from build123d import *

# Parameters (mm, degrees)
SKETCH1_W           = 102
SKETCH1_H           = 85
BOSS_EXTRUDE1_DEPTH = 38
SKETCH2_R           = 2.1
CUT_EXTRUDE1_DEPTH  = 35
SKETCH3_R           = 2.1
CUT_EXTRUDE2_DEPTH  = 35
SKETCH5_R           = 4
CUT_EXTRUDE4_DEPTH  = 10
FILLET1_R           = 5
FILLET2_R           = 5
FILLET3_R           = 5
FILLET4_R           = 5
SKETCH6_R           = 1.6
BOSS_EXTRUDE2_DEPTH = 5
SKETCH7_W           = 15
SKETCH7_H           = 4
BOSS_EXTRUDE3_DEPTH = 12
CHAMFER1_SIZE       = 5
CHAMFER2_SIZE       = 5
SKETCH8_R           = 3.012300636
CUT_EXTRUDE5_DEPTH  = 5
FILLET5_R           = 2
FILLET6_R           = 2
FILLET7_R           = 2
FILLET8_R           = 2
SKETCH9_W           = 1
SKETCH9_H           = 10
CUT_EXTRUDE6_DEPTH  = 2.1
SKETCH10_W          = 1
SKETCH10_H          = 10
CUT_EXTRUDE7_DEPTH  = 2.1


with BuildPart() as part:
    # Sketch1 → Boss-Extrude1 (new body)
    with BuildSketch(Plane(origin=(0, 0, 0), x_dir=(1, 0, 0), z_dir=(0, 1, 0))):
        Rectangle(SKETCH1_W, SKETCH1_H)
    extrude(amount=BOSS_EXTRUDE1_DEPTH)

    # Sketch2 → Cut-Extrude1 (cut)
    with BuildSketch(Plane(origin=(0, 38, 0), x_dir=(1, 0, 0), z_dir=(0, 1, 0))):
        with Locations((43, 34.5)):
            Circle(SKETCH2_R)
        with Locations((-43, -34.5)):
            Circle(SKETCH2_R)
        with Locations((43, -34.5)):
            Circle(SKETCH2_R)
        Polygon((-39, 40.5), (39, 40.5), (39, 30.5), (49, 30.5), (49, -30.5), (39, -30.5), (39, -40.5), (-39, -40.5), (-39, -30.5), (-49, -30.5), (-49, 30.5), (-39, 30.5), align=None)
    extrude(amount=-CUT_EXTRUDE1_DEPTH, mode=Mode.SUBTRACT)

    # Sketch3 → Cut-Extrude2 (cut)
    with BuildSketch(Plane(origin=(0, 38, 0), x_dir=(1, 0, 0), z_dir=(0, 1, 0))):
        with Locations((-43, 34.5)):
            Circle(SKETCH3_R)
    extrude(amount=-CUT_EXTRUDE2_DEPTH, mode=Mode.SUBTRACT)

    # Sketch5 → Cut-Extrude4 (cut)
    with BuildSketch(Plane.ZY.offset(51)):
        with Locations((-17.5, 7.998461061)):
            Circle(SKETCH5_R)
        with Locations((17.5, 7.998461061)):
            Circle(SKETCH5_R)
    extrude(amount=-CUT_EXTRUDE4_DEPTH, mode=Mode.SUBTRACT)

    # Fillet1
    fillet1_edges = [part.edges().sort_by_distance(p)[0] for p in [
        (-51, 19, 42.5),
    ]]
    fillet(fillet1_edges, radius=FILLET1_R)

    # Fillet2
    fillet2_edges = [part.edges().sort_by_distance(p)[0] for p in [
        (-51, 19, -42.5),
    ]]
    fillet(fillet2_edges, radius=FILLET2_R)

    # Fillet3
    fillet3_edges = [part.edges().sort_by_distance(p)[0] for p in [
        (51, 19, 42.5),
    ]]
    fillet(fillet3_edges, radius=FILLET3_R)

    # Fillet4
    fillet4_edges = [part.edges().sort_by_distance(p)[0] for p in [
        (51, 19, -42.5),
    ]]
    fillet(fillet4_edges, radius=FILLET4_R)

    # Sketch6 → Boss-Extrude2 (add)
    with BuildSketch(Plane(origin=(0, 3, 0), x_dir=(1, 0, 0), z_dir=(0, 1, 0))):
        with Locations((-33.5, 26.565019739)):
            Circle(SKETCH6_R)
        with Locations((-33.5, -5.434980261)):
            Circle(SKETCH6_R)
        with Locations((33.5, 26.565019739)):
            Circle(SKETCH6_R)
        with Locations((33.5, -5.434980261)):
            Circle(SKETCH6_R)
    extrude(amount=BOSS_EXTRUDE2_DEPTH)

    # Sketch7 → Boss-Extrude3 (add)
    with BuildSketch(Plane.ZY.offset(51)):
        with Locations((0, 2)):
            Rectangle(SKETCH7_W, SKETCH7_H)
    extrude(amount=BOSS_EXTRUDE3_DEPTH)

    # Chamfer1
    chamfer1_edges = [part.edges().sort_by_distance(p)[0] for p in [
        (-63, 2, -7.5),
    ]]
    chamfer(chamfer1_edges, length=CHAMFER1_SIZE)

    # Chamfer2
    chamfer2_edges = [part.edges().sort_by_distance(p)[0] for p in [
        (-63, 2, 7.5),
    ]]
    chamfer(chamfer2_edges, length=CHAMFER2_SIZE)

    # Sketch8 → Cut-Extrude5 (cut)
    with BuildSketch(Plane(origin=(0, 4, 0), x_dir=(1, 0, 0), z_dir=(0, 1, 0))):
        with Locations((-56.61368814, 0)):
            Circle(SKETCH8_R)
    extrude(amount=-CUT_EXTRUDE5_DEPTH, mode=Mode.SUBTRACT)

    # Fillet5
    fillet5_edges = [part.edges().sort_by_distance(p)[0] for p in [
        (-58, 2, -7.5),
    ]]
    fillet(fillet5_edges, radius=FILLET5_R)

    # Fillet6
    fillet6_edges = [part.edges().sort_by_distance(p)[0] for p in [
        (-63, 2, -2.5),
    ]]
    fillet(fillet6_edges, radius=FILLET6_R)

    # Fillet7
    fillet7_edges = [part.edges().sort_by_distance(p)[0] for p in [
        (-63, 2, 2.5),
    ]]
    fillet(fillet7_edges, radius=FILLET7_R)

    # Fillet8
    fillet8_edges = [part.edges().sort_by_distance(p)[0] for p in [
        (-58, 2, 7.5),
    ]]
    fillet(fillet8_edges, radius=FILLET8_R)

    # Sketch9 → Cut-Extrude6 (cut)
    with BuildSketch(Plane.XY.offset(42.5)):
        with Locations((-30.5, 28)):
            Rectangle(SKETCH9_W, SKETCH9_H)
    extrude(amount=-CUT_EXTRUDE6_DEPTH, mode=Mode.SUBTRACT)

    # Sketch10 → Cut-Extrude7 (cut)
    with BuildSketch(Plane.XY.offset(42.5)):
        with Locations((-27.5, 28)):
            Rectangle(SKETCH10_W, SKETCH10_H)
        with Locations((-24.5, 28)):
            Rectangle(SKETCH10_W, SKETCH10_H)
        with Locations((-21.5, 28)):
            Rectangle(SKETCH10_W, SKETCH10_H)
    extrude(amount=-CUT_EXTRUDE7_DEPTH, mode=Mode.SUBTRACT)


solid = part.part
Check sheet for the modelled part. Datum: model origin and axes. Units: mm. A direction names the side the tool comes from. Round coordinates to 2 decimals unless told otherwise and drop trailing zeros. Loops run counter-clockwise (first coordinate to the right, second up) from the corner with the lowest first, then second, coordinate; pieces in that order, holes last.
1. Sectioned sample at D-D on z = 34.5. Record the boundary of the cut face in (x, y).
2. Sectioned sample at C-C on x = -33.5. Record the boundary of the cut face in (y, z).
3. Sectioned sample at B-B on y = 18.5. Record the boundary of the cut face in (x, z), and give its area (3 significant figures).
4. Gauge pin test, flat ends, axial feed: pin 1 Ø3.5 at (x, z) = (-56.5, 0) entering from +Y; pin 2 Ø1.6 at (y, z) = (28, 41.5) entering from +X; pin 3 Ø2 at (x, z) = (-23, 3) entering from -Y; pin 4 Ø1 at (y, z) = (32, -26.5) entering from -X. Record the tip position at first contact, or that the pin passes through.
5. Sectioned sample at A-A on z = 17.5. Record the boundary of the cut face in (x, y).
6. Mould release check, pull along X, two halves, no side actions. Record for faces 4 (the flat face through (-43, 3, -35)), 5 (the flat face through (-63, 2, 0)), 6 (the flat face through (-49.3, 38, -0.2)): released by +X, released by -X, zero draft, split by the parting line, or undercut.
7. Scan lines: probe 1 along Z at (x, y) = (-43, 22); probe 2 along X at (y, z) = (26, 34.5); probe 3 along Z at (x, y) = (19, 8). Record each from-to range of solid material in increasing order.
8. Set-up check for faces 1 (the flat face through (-60.5, 2, 5)), 2 (the flat face through (-44, 21, -30.5)), 3 (the cylindrical face through (-50.014, 8.174, -21.496)): record each of +Z, -Z, +X, -X, +Y, -Y from which the full face is reachable in a straight line by a thin tool's end or side.
Recorded:
1. outline: (-51, 0) - (51, 0) - (51, 38) - (45.1, 38) - (45.1, 3) - (40.9, 3) - (40.9, 38) - (39, 38) - (39, 3) - (-39, 3) - (-39, 38) - (-40.9, 38) - (-40.9, 3) - (-45.1, 3) - (-45.1, 38) - (-51, 38) - close
2. outline: (0, -42.5) - (38, -42.5) - (38, -40.5) - (3, -40.5) - (3, -28.17) - (8, -28.17) - (8, -24.97) - (3, -24.97) - (3, 3.83) - (8, 3.83) - (8, 7.03) - (3, 7.03) - (3, 40.5) - (38, 40.5) - (38, 42.5) - (0, 42.5) - close
3. outline: (-51, -37.5) arc R5 ccw to (-46, -42.5) - (46, -42.5) arc R5 ccw to (51, -37.5) - (51, 37.5) arc R5 ccw to (46, 42.5) - (-46, 42.5) arc R5 ccw to (-51, 37.5) - close; hole (-49, -30.5) - (-39, -30.5) - (-39, -40.5) - (39, -40.5) - (39, -30.5) - (49, -30.5) - (49, 30.5) - (39, 30.5) - (39, 40.5) - (-39, 40.5) - (-39, 30.5) - (-49, 30.5) - close; hole circle Ø4.2 at (-43, -34.5); hole circle Ø4.2 at (-43, 34.5); hole circle Ø4.2 at (43, -34.5); hole circle Ø4.2 at (43, 34.5)
3. area: 1,060 mm2
4. pin 1: passes through
4. pin 2: stops at x = 49.84
4. pin 3: stops at y = 0
4. pin 4: stops at x = -51
5. outline: (-51, 0) - (51, 0) - (51, 38) - (49, 38) - (49, 3) - (-49, 3) - (-49, 4) - (-51, 4) - close; (-51, 12) - (-49, 12) - (-49, 38) - (-51, 38) - close
6. face 4: undercut
6. face 5: released by -X
6. face 6: zero draft
7. probe 1: z = -42.5 to -36.6, -32.4 to -30.5, 30.5 to 32.4, 36.6 to 42.5
7. probe 2: x = -51 to -45.1, -40.9 to -39, 39 to 40.9, 45.1 to 51
7. probe 3: z = -42.5 to -40.5, 40.5 to 42.5
8. face 1: +Z, -X, +Y, -Y
8. face 2: +Y
8. face 3: -X
